For this review, take the finished solid that the model builds, in its own axes (mm). A direction names the side the tool comes from. Coordinates: 2 decimals unless noted, no trailing zeros. Write each loop counter-clockwise with the first axis right and the second up, starting at its lowest first coordinate (ties: lowest second). Pieces come first, ordered by that corner, then holes. Notation, with made-up numbers: (81.5, 6) -> (126.5, 6) arc R34 cw to (126.5, 43) -> close; hole circle Ø8 at (-12.75, 55). An arc over 180 degrees is marked (long way). Put each result on its own line as item: value. Start each with the question number.
Item 1: Consider section D-D on y = -5. Give the boundary of the cut face in (x, z) (3 decimals), and give its area (3 significant figures).
Item 2: To check wall thickness, follow L1, parallel to X at y = 0.8, z = 12.25; L2, parallel to Z at x = 12.25, y = 2.7. State the ranges of each line that lie inside material, in increasing order.
Item 3: Consider section A-A on x = 0. Give the boundary of the cut face in (y, z), and give its area (3 significant figures).
Item 4: Consider section B-B on z = -8. Give the boundary of the cut face in (x, y), and give its area (3 significant figures).
Item 5: Insertion check: P1, Ø8, axis at x = -7.5, y = -5, coming from the +Z side; P2, Ø1.2, axis at x = -12.25, z = 12.25, coming from the -Y side; P3, Ø1.5, axis at x = 17, z = 14, coming from the -Y side; P4, Ø1.4, axis at x = 12.25, z = -12.25, coming from the +Y side. Each pin has a flat end and moves straight along its axis. Give the tip position at first contact, or say it passes through.
Item 6: Consider section C-C on z = 12.25. Give the boundary of the cut face in (x, y), and give its area (3 significant figures).
Item 7: For faces 1 (the cylindrical face through (11.7, 1.97, -12.76)), 2 (the flat face through (0, -5, -11)), 3 (the flat face through (3.75, 2, 11)), 4 (the flat face through (15.5, -5, 14)), list the 3-axis set-ups (+Z, -Z, +X, -X, +Y, -Y) from which the entire face can be reached by the end or side of a thin tool; tool diameter is ignored.
Item 8: The part is to be moulded in two halves that separate along X. For faces 5 (the flat face through (15.5, 0.2, -5.2)), 6 (the flat face through (-7, 0, 8)), 7 (the cylindrical face through (11.302, -3.902, -13.218)), 8 (the flat face through (-0.3, 0.3, 15.5)), say which applies: +X half, -X half, draft (parallel to the pull), parting line (faces both ways), or undercut.
```python
from build123d import *

# Parameters (mm, degrees)
SKETCH1_W           = 31
SKETCH1_H           = 31
SKETCH1_R           = 0.75
SKETCH1_R_2         = 10
BOSS_EXTRUDE1_DEPTH = 4
SKETCH2_W           = 31
SKETCH2_H           = 4.5
BOSS_EXTRUDE2_DEPTH = 10
SKETCH3_R           = 1.625
CUT_EXTRUDE1_DEPTH  = 5.5
SKETCH4_W           = 7.5
SKETCH4_H           = 8
CUT_EXTRUDE2_DEPTH  = 15
SKETCH5_R           = 20
CUT_EXTRUDE3_DEPTH  = 0.5
SKETCH6_W           = 3
SKETCH6_H           = 4
BOSS_EXTRUDE3_DEPTH = 13.5


with BuildPart() as part:
    # Sketch1 → Boss-Extrude1 (new body)
    with BuildSketch(Plane(origin=(0, 0, 0), x_dir=(1, 0, 0), z_dir=(0, 1, 0))):
        Rectangle(SKETCH1_W, SKETCH1_H)
        with Locations((-12.25, 12.25)):
            Circle(SKETCH1_R, mode=Mode.SUBTRACT)
        with Locations((12.25, 12.25)):
            Circle(SKETCH1_R, mode=Mode.SUBTRACT)
        with Locations((12.25, -12.25)):
            Circle(SKETCH1_R, mode=Mode.SUBTRACT)
        with Locations((-12.25, -12.25)):
            Circle(SKETCH1_R, mode=Mode.SUBTRACT)
        Circle(SKETCH1_R_2, mode=Mode.SUBTRACT)
    extrude(amount=BOSS_EXTRUDE1_DEPTH)

    # Sketch2 → Boss-Extrude2 (add)
    with BuildSketch(Plane.XZ):
        with Locations((0, -13.25)):
            Rectangle(SKETCH2_W, SKETCH2_H)
    extrude(amount=BOSS_EXTRUDE2_DEPTH)

    # Sketch3 → Cut-Extrude1 (cut, through all)
    with BuildSketch(Plane.XY.offset(-11)):
        with Locations((-12.5, -5)):
            Circle(SKETCH3_R)
        with Locations((12.5, -5)):
            Circle(SKETCH3_R)
    extrude(amount=-CUT_EXTRUDE1_DEPTH, mode=Mode.SUBTRACT)

    # Sketch4 → Cut-Extrude2 (cut, through all)
    with BuildSketch(Plane(origin=(0, 4, 0), x_dir=(1, 0, 0), z_dir=(0, 1, 0))):
        with Locations((0, -9)):
            Rectangle(SKETCH4_W, SKETCH4_H)
    extrude(amount=-CUT_EXTRUDE2_DEPTH, mode=Mode.SUBTRACT)

    # Sketch5 → Cut-Extrude3 (cut)
    with BuildSketch(Plane.XZ.offset(10)):
        with Locations((0, 5)):
            Circle(SKETCH5_R)
    extrude(amount=-CUT_EXTRUDE3_DEPTH, mode=Mode.SUBTRACT)

    # Sketch6 → Boss-Extrude3 (add)
    with BuildSketch(Plane(origin=(0, 4, 0), x_dir=(1, 0, 0), z_dir=(0, 1, 0))):
        with Locations((-17, -13.5)):
            Rectangle(SKETCH6_W, SKETCH6_H)
        with Locations((17, -13.5)):
            Rectangle(SKETCH6_W, SKETCH6_H)
    extrude(amount=-BOSS_EXTRUDE3_DEPTH)


solid = part.part
```
Return value:
1. outline: (-18.5, 11.5) -> (-15.5, 11.5) -> (-15.5, 15.5) -> (-18.5, 15.5) -> close; (-15.5, -15.5) -> (-14.125, -15.5) -> (-14.125, -11) -> (-15.5, -11) -> close; (-10.875, -15.5) -> (10.875, -15.5) -> (10.875, -11) -> (-10.875, -11) -> close; (14.125, -15.5) -> (15.5, -15.5) -> (15.5, -11) -> (14.125, -11) -> close; (15.5, 11.5) -> (18.5, 11.5) -> (18.5, 15.5) -> (15.5, 15.5) -> close
1. area: 134 mm^2
2. L1: -18.5 to -13, -11.5 to -3.75, 3.75 to 11.5, 13 to 18.5
2. L2: -15.5 to -13, -11.5 to 11.5, 13 to 15.5
3. outline: (-10, -15.5) -> (4, -15.5) -> (4, -10) -> (0, -10) -> (0, -11) -> (-9.5, -11) -> (-9.5, -15) -> (-10, -15) -> close; (0, 13) -> (4, 13) -> (4, 15.5) -> (0, 15.5) -> close
3. area: 75.0 mm^2
4. outline: (-15.5, 0) -> (-6, 0) -> (-6, 4) -> (-15.5, 4) -> close; (6, 0) -> (15.5, 0) -> (15.5, 4) -> (6, 4) -> close
4. area: 76.0 mm^2
5. P1: z = -11
5. P2: through
5. P3: y = -9.5
5. P4: y = 0
6. outline: (-18.5, -9.5) -> (-15.5, -9.5) -> (-15.5, 0) -> (-13, 0) -> (-13, 4) -> (-18.5, 4) -> close; (-11.5, 0) -> (-3.75, 0) -> (-3.75, 4) -> (-11.5, 4) -> close; (3.75, 0) -> (11.5, 0) -> (11.5, 4) -> (3.75, 4) -> close; (13, 0) -> (15.5, 0) -> (15.5, -9.5) -> (18.5, -9.5) -> (18.5, 4) -> (13, 4) -> close
6. area: 163 mm^2
7. face 1: +Y
7. face 2: +Z, +X, -X, -Y
7. face 3: +Y, -Y
7. face 4: +Z, -Y
8. face 5: +X half
8. face 6: undercut
8. face 7: undercut
8. face 8: draft
